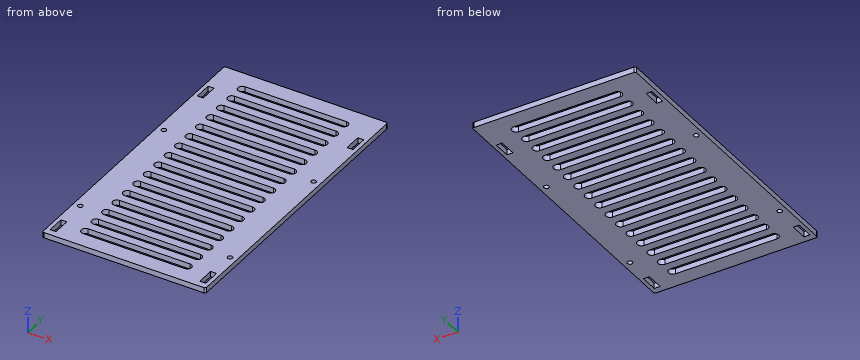
```python
from build123d import *

# Parameters (mm, degrees)
STOCK_TORSO_REAR_PLATE_1_START       = -1.5875
STOCK_TORSO_REAR_PLATE_1_OUTLINE_W   = 96.34
STOCK_TORSO_REAR_PLATE_1_OUTLINE_H   = 174.5
STOCK_TORSO_REAR_PLATE_1_OUTLINE_W_2 = 3.4925
STOCK_TORSO_REAR_PLATE_1_OUTLINE_H_2 = 10.25
STOCK_TORSO_REAR_PLATE_1_OUTLINE_R   = 1.45
STOCK_TORSO_REAR_PLATE_1_DEPTH       = 3.175
FILLET1_R                            = 1


# Read off the part's stored shape, not the designer's step: Stock-torso_rear_plate-1
with BuildPart() as part:
    # Stock-torso_rear_plate-1 outline → Stock-torso_rear_plate-1 (new body)
    with BuildSketch(Plane.XY.offset(STOCK_TORSO_REAR_PLATE_1_START)):
        with Locations((0, -62.75)):
            Rectangle(STOCK_TORSO_REAR_PLATE_1_OUTLINE_W, STOCK_TORSO_REAR_PLATE_1_OUTLINE_H)
        with Locations((-44.17, -141)):
            Rectangle(STOCK_TORSO_REAR_PLATE_1_OUTLINE_W_2, STOCK_TORSO_REAR_PLATE_1_OUTLINE_H_2, mode=Mode.SUBTRACT)
        with Locations((-44.17, -120)):
            Circle(STOCK_TORSO_REAR_PLATE_1_OUTLINE_R, mode=Mode.SUBTRACT)
        with BuildLine():
            Line((30, -140.5), (-30, -140.5))
            ThreePointArc((-30, -140.5), (-32.5, -138), (-30, -135.5))
            Line((-30, -135.5), (30, -135.5))
            ThreePointArc((30, -135.5), (32.5, -138), (30, -140.5))
        make_face(mode=Mode.SUBTRACT)
        with BuildLine():
            Line((30, -130.5), (-30, -130.5))
            ThreePointArc((-30, -130.5), (-32.5, -128), (-30, -125.5))
            Line((-30, -125.5), (30, -125.5))
            ThreePointArc((30, -125.5), (32.5, -128), (30, -130.5))
        make_face(mode=Mode.SUBTRACT)
        with BuildLine():
            Line((30, -120.5), (-30, -120.5))
            ThreePointArc((-30, -120.5), (-32.5, -118), (-30, -115.5))
            Line((-30, -115.5), (30, -115.5))
            ThreePointArc((30, -115.5), (32.5, -118), (30, -120.5))
        make_face(mode=Mode.SUBTRACT)
        with BuildLine():
            Line((30, -110.5), (-30, -110.5))
            ThreePointArc((-30, -110.5), (-32.5, -108), (-30, -105.5))
            Line((-30, -105.5), (30, -105.5))
            ThreePointArc((30, -105.5), (32.5, -108), (30, -110.5))
        make_face(mode=Mode.SUBTRACT)
        with Locations((44.17, -141)):
            Rectangle(STOCK_TORSO_REAR_PLATE_1_OUTLINE_W_2, STOCK_TORSO_REAR_PLATE_1_OUTLINE_H_2, mode=Mode.SUBTRACT)
        with Locations((44.17, -120)):
            Circle(STOCK_TORSO_REAR_PLATE_1_OUTLINE_R, mode=Mode.SUBTRACT)
        with BuildLine():
            Line((30, -100.5), (-30, -100.5))
            ThreePointArc((-30, -100.5), (-32.5, -98), (-30, -95.5))
            Line((-30, -95.5), (30, -95.5))
            ThreePointArc((30, -95.5), (32.5, -98), (30, -100.5))
        make_face(mode=Mode.SUBTRACT)
        with BuildLine():
            Line((30, -90.5), (-30, -90.5))
            ThreePointArc((-30, -90.5), (-32.5, -88), (-30, -85.5))
            Line((-30, -85.5), (30, -85.5))
            ThreePointArc((30, -85.5), (32.5, -88), (30, -90.5))
        make_face(mode=Mode.SUBTRACT)
        with BuildLine():
            Line((30, -80.5), (-30, -80.5))
            ThreePointArc((-30, -80.5), (-32.5, -78), (-30, -75.5))
            Line((-30, -75.5), (30, -75.5))
            ThreePointArc((30, -75.5), (32.5, -78), (30, -80.5))
        make_face(mode=Mode.SUBTRACT)
        with BuildLine():
            Line((30, -70.5), (-30, -70.5))
            ThreePointArc((-30, -70.5), (-32.5, -68), (-30, -65.5))
            Line((-30, -65.5), (30, -65.5))
            ThreePointArc((30, -65.5), (32.5, -68), (30, -70.5))
        make_face(mode=Mode.SUBTRACT)
        with Locations((-44.17, -40)):
            Circle(STOCK_TORSO_REAR_PLATE_1_OUTLINE_R, mode=Mode.SUBTRACT)
        with Locations((-44.17, 0)):
            Rectangle(STOCK_TORSO_REAR_PLATE_1_OUTLINE_W_2, STOCK_TORSO_REAR_PLATE_1_OUTLINE_H_2, mode=Mode.SUBTRACT)
        with BuildLine():
            Line((30, -60.5), (-30, -60.5))
            ThreePointArc((-30, -60.5), (-32.5, -58), (-30, -55.5))
            Line((-30, -55.5), (30, -55.5))
            ThreePointArc((30, -55.5), (32.5, -58), (30, -60.5))
        make_face(mode=Mode.SUBTRACT)
        with BuildLine():
            Line((30, -50.5), (-30, -50.5))
            ThreePointArc((-30, -50.5), (-32.5, -48), (-30, -45.5))
            Line((-30, -45.5), (30, -45.5))
            ThreePointArc((30, -45.5), (32.5, -48), (30, -50.5))
        make_face(mode=Mode.SUBTRACT)
        with BuildLine():
            Line((30, -40.5), (-30, -40.5))
            ThreePointArc((-30, -40.5), (-32.5, -38), (-30, -35.5))
            Line((-30, -35.5), (30, -35.5))
            ThreePointArc((30, -35.5), (32.5, -38), (30, -40.5))
        make_face(mode=Mode.SUBTRACT)
        with BuildLine():
            Line((30, -30.5), (-30, -30.5))
            ThreePointArc((-30, -30.5), (-32.5, -28), (-30, -25.5))
            Line((-30, -25.5), (30, -25.5))
            ThreePointArc((30, -25.5), (32.5, -28), (30, -30.5))
        make_face(mode=Mode.SUBTRACT)
        with Locations((44.17, -40)):
            Circle(STOCK_TORSO_REAR_PLATE_1_OUTLINE_R, mode=Mode.SUBTRACT)
        with BuildLine():
            Line((30, -20.5), (-30, -20.5))
            ThreePointArc((-30, -20.5), (-32.5, -18), (-30, -15.5))
            Line((-30, -15.5), (30, -15.5))
            ThreePointArc((30, -15.5), (32.5, -18), (30, -20.5))
        make_face(mode=Mode.SUBTRACT)
        with BuildLine():
            Line((30, -10.5), (-30, -10.5))
            ThreePointArc((-30, -10.5), (-32.5, -8), (-30, -5.5))
            Line((-30, -5.5), (30, -5.5))
            ThreePointArc((30, -5.5), (32.5, -8), (30, -10.5))
        make_face(mode=Mode.SUBTRACT)
        with BuildLine():
            Line((-30, 4.5), (30, 4.5))
            ThreePointArc((30, 4.5), (32.5, 2), (30, -0.5))
            Line((30, -0.5), (-30, -0.5))
            ThreePointArc((-30, -0.5), (-32.5, 2), (-30, 4.5))
        make_face(mode=Mode.SUBTRACT)
        with BuildLine():
            Line((-30, 14.5), (30, 14.5))
            ThreePointArc((30, 14.5), (32.5, 12), (30, 9.5))
            Line((30, 9.5), (-30, 9.5))
            ThreePointArc((-30, 9.5), (-32.5, 12), (-30, 14.5))
        make_face(mode=Mode.SUBTRACT)
        with Locations((44.17, 0)):
            Rectangle(STOCK_TORSO_REAR_PLATE_1_OUTLINE_W_2, STOCK_TORSO_REAR_PLATE_1_OUTLINE_H_2, mode=Mode.SUBTRACT)
    extrude(amount=STOCK_TORSO_REAR_PLATE_1_DEPTH)

    # Fillet1
    fillet1_edges = [part.edges().sort_by_distance(p)[0] for p in [
        (-48.17, 24.5, 0),
        (48.17, 24.5, 0),
        (48.17, -150, 0),
        (-48.17, -150, 0),
    ]]
    fillet(fillet1_edges, radius=FILLET1_R)


solid = part.part
```
The listing builds one solid part. Answer for the finished solid, in the listing's coordinates (mm). Round coordinates to 2 decimals unless told otherwise and drop trailing zeros. Write each loop counter-clockwise with the first axis right and the second up, starting at its lowest first coordinate (ties: lowest second). Pieces come first, ordered by that corner, then holes. Notation, with made-up numbers: (3, 64.5) -> (18, 64.5) arc R24 ccw to (18, 83.5) -> close; hole circle Ø6 at (52.5, 45.5). An arc over 180 degrees is marked (long way). Answer as a JSON object with one key per item and string values. Group by question number.
Q1. Section C-C (x = 2) is taken. Count the separate pieces of the cut face and the enclosed holes in it, plus the area to 3 significant figures.
Q2. Section A-A (y = -98) is taken. Write down the section's boundary in (x, z), plus the area to 3 significant figures.
Q3. Section B-B (y = -138) is taken. Write down the section's boundary in (x, z), plus the area to 3 significant figures.
Q4. Straight lines are drawn through the part: line 1 along Y through (x, z) = (44.17, 0.6) (3 decimals); line 2 along X through (y, z) = (-1.5, -0.8); line 3 along X through (y, z) = (-28, -1). For each, find the intervals that lie inside material, in ascending order.
Check values:
{
 "1": {"separate pieces": "17", "enclosed holes": "0", "area": "300 mm^2"},
 "2": {"outline": "(-48.17, -1.59) -> (-32.5, -1.59) -> (-32.5, 1.59) -> (-48.17, 1.59) -> close; (32.5, -1.59) -> (48.17, -1.59) -> (48.17, 1.59) -> (32.5, 1.59) -> close", "area": "99.5 mm^2"},
 "3": {"outline": "(-48.17, -1.59) -> (-45.92, -1.59) -> (-45.92, 1.59) -> (-48.17, 1.59) -> close; (-42.42, -1.59) -> (-32.5, -1.59) -> (-32.5, 1.59) -> (-42.42, 1.59) -> close; (32.5, -1.59) -> (42.42, -1.59) -> (42.42, 1.59) -> (32.5, 1.59) -> close; (45.92, -1.59) -> (48.17, -1.59) -> (48.17, 1.59) -> (45.92, 1.59) -> close", "area": "77.3 mm^2"},
 "4": {"line 1": "-150 to -146.125, -135.875 to -121.45, -118.55 to -41.45, -38.55 to -5.125, 5.125 to 24.5", "line 2": "-48.17 to -45.92, -42.42 to 42.42, 45.92 to 48.17", "line 3": "-48.17 to -32.5, 32.5 to 48.17"}
}
